Geometry check sheet. Reference: the model listing, model coordinates, mm. A direction names the side the tool comes from. Give positions to 0.01 mm unless a question says otherwise; leave off trailing zeros. Write each loop counter-clockwise with the first axis right and the second up, starting at its lowest first coordinate (ties: lowest second). Pieces come first, ordered by that corner, then holes. Notation, with made-up numbers: (84, 49) -> (134, 49) arc R10 ccw to (134, 56) -> close; hole circle Ø9 at (-1.75, 7). An arc over 180 degrees is marked (long way). One line per item, written item: value.
from build123d import *

# Parameters (mm, degrees)
SKETCH1_R           = 7
BOSS_EXTRUDE1_DEPTH = 320
SKETCH2_R           = 10
BOSS_EXTRUDE2_DEPTH = 10
BOSS_EXTRUDE3_START = -10
SKETCH3_R           = 10
BOSS_EXTRUDE3_DEPTH = 10


with BuildPart() as part:
    # Sketch1 → Boss-Extrude1 (new body)
    with BuildSketch(Plane.XY):
        Circle(SKETCH1_R)
    extrude(amount=BOSS_EXTRUDE1_DEPTH)

    # Sketch2 → Boss-Extrude2 (add)
    with BuildSketch(Plane.XY.offset(320)):
        Circle(SKETCH2_R)
    extrude(amount=-BOSS_EXTRUDE2_DEPTH)

    # Sketch3 → Boss-Extrude3 (add)
    with BuildSketch(Plane(origin=(0, 0, 0), x_dir=(-1, 0, 0), z_dir=(0, 0, -1)).offset(BOSS_EXTRUDE3_START)):
        with Locations(Location((0, 0, 0), (0, 0, 180))):
            Circle(SKETCH3_R)
    extrude(amount=BOSS_EXTRUDE3_DEPTH)


solid = part.part
1) Depth check by flat-ended pin: pin 1 Ø10 at (x, z) = (-5.5, 211) entering from +Y; pin 2 Ø8 at (y, z) = (0.5, 76.5) entering from -X; pin 3 Ø12 at (y, z) = (-2, 104.5) entering from +X. Enter the tip coordinate at first touch or a pass-through.
Verdict:
pin 1: y = 6.98
pin 2: x = -7
pin 3: x = 7
2) Scan lines: probe 1 along Z at (x, y) = (8.5, 2.75); probe 2 along X at (y, z) = (0.75, 200.5); probe 3 along X at (y, z) = (-5, 79). Record each from-to range of solid material in increasing order.
Verdict:
probe 1: 0 to 10, 310 to 320
probe 2: -6.96 to 6.96
probe 3: -4.9 to 4.9
3) Sectioned sample at C-C on z = 218. Record the cut outline in (x, y).
Verdict:
outline: circle Ø14 at (0, 0)
4) Sectioned sample at A-A on y = 0. Record the cut outline in (x, z).
Verdict:
outline: (-10, 0) -> (10, 0) -> (10, 10) -> (7, 10) -> (7, 310) -> (10, 310) -> (10, 320) -> (-10, 320) -> (-10, 310) -> (-7, 310) -> (-7, 10) -> (-10, 10) -> close
5) Tool access check on faces 4 (the cylindrical face through (6.466, -2.681, 157.9)), 5 (the cylindrical face through (-2.17, -9.76, 315.07)). Record the directions out of +Z, -Z, +X, -X, +Y, -Y that give a thin tool (end or side, any length) a straight path to the whole face; none if there is none.
Verdict:
face 4: none
face 5: +Z, -Z
6) Mould release check, pull along Z, two halves, no side actions. Record for faces 1 (the cylindrical face through (-10, 0, 5)), 2 (the flat face through (0, 0, 320)), 3 (the flat face through (-7, -2, 310)): released by +Z, released by -Z, zero draft, split by the parting line, or undercut.
Verdict:
face 1: zero draft
face 2: released by +Z
face 3: undercut
